```python
from build123d import *

# Parameters (mm, degrees)
SKETCH1_W                 = 79.1
SKETCH1_H                 = 60
BOSS_EXTRUDE1_DEPTH       = 5
BOSS_EXTRUDE2_DEPTH       = 24
MIRROR2_COPY_1_DEPTH      = 24
SKETCH9_W                 = 10
SKETCH9_H                 = 9.8
SKETCH9_W_2               = 6
SKETCH9_H_2               = 2.8
BOSS_EXTRUDE4_DEPTH       = 8
MIRROR9_COPY_1_SKETCH_W   = 10
MIRROR9_COPY_1_SKETCH_H   = 9.8
MIRROR9_COPY_1_SKETCH_W_2 = 6
MIRROR9_COPY_1_SKETCH_H_2 = 2.8
MIRROR9_COPY_1_DEPTH      = 8
SKETCH10_R                = 1.55
CUT_EXTRUDE6_DEPTH        = 15.8
SKETCH11_W                = 79.1
SKETCH11_H                = 16
BOSS_EXTRUDE5_DEPTH       = 16
SKETCH12_R                = 4.05
CUT_EXTRUDE7_DEPTH        = 80.1
SKETCH13_W                = 6
SKETCH13_H                = 2.8
CUT_EXTRUDE8_DEPTH        = 61
SKETCH14_R                = 1.55
CUT_EXTRUDE9_DEPTH        = 10
SKETCH14_3_W              = 6
SKETCH14_3_H              = 35
CUT_EXTRUDE10_DEPTH       = 4.8
FILLET1_R                 = 8
SKETCH15_W                = 50.3
SKETCH15_H                = 42.3
SKETCH15_R                = 1.55
SKETCH15_R_2              = 12.5
BOSS_EXTRUDE6_DEPTH       = 5
FILLET3_R                 = 3


with BuildPart() as part:
    # Sketch1 → Boss-Extrude1 (new body)
    with BuildSketch(Plane(origin=(0, 0, 0), x_dir=(1, 0, 0), z_dir=(0, 1, 0))):
        Rectangle(SKETCH1_W, SKETCH1_H)
    extrude(amount=BOSS_EXTRUDE1_DEPTH)

    # Sketch2 → Boss-Extrude2 (add)
    with BuildSketch(Plane.XY.offset(30)):
        with BuildLine():
            Line((-39.55, 13.55), (-39.55, 5))
            Line((-39.55, 5), (-20.45, 5))
            Line((-20.45, 5), (-20.45, 13.55))
            Line((-20.45, 13.55), (-22.45, 13.55))
            ThreePointArc((-22.45, 13.55), (-30, 6), (-37.55, 13.55))
            Line((-37.55, 13.55), (-39.55, 13.55))
        make_face()
    boss_extrude2 = extrude(amount=-BOSS_EXTRUDE2_DEPTH)

    # Mirror1: Boss-Extrude2 across plane
    add(boss_extrude2.mirror(Plane.XY))

    # Mirror2: Boss-Extrude2 across plane
    add(boss_extrude2.mirror(Plane(origin=(0, 0, 0), x_dir=(0, 0, 1), z_dir=(1, 0, 0))))

    # Mirror2 copy 1 sketch → Mirror2 copy 1 (add)
    with BuildSketch(Plane(origin=(0, 0, -30), x_dir=(-1, 0, 0), z_dir=(0, 0, -1))):
        with BuildLine():
            Line((-39.55, 13.55), (-39.55, 5))
            Line((-39.55, 5), (-20.45, 5))
            Line((-20.45, 5), (-20.45, 13.55))
            Line((-20.45, 13.55), (-22.45, 13.55))
            ThreePointArc((-22.45, 13.55), (-30, 6), (-37.55, 13.55))
            Line((-37.55, 13.55), (-39.55, 13.55))
        make_face()
    extrude(amount=-MIRROR2_COPY_1_DEPTH)

    # Sketch9 → Boss-Extrude4 (add)
    with BuildSketch(Plane.XY.offset(30)):
        with Locations((-15.45, 9.9)):
            Rectangle(SKETCH9_W, SKETCH9_H)
        with Locations((-15.45, 9.4)):
            Rectangle(SKETCH9_W_2, SKETCH9_H_2, mode=Mode.SUBTRACT)
    boss_extrude4 = extrude(amount=-BOSS_EXTRUDE4_DEPTH)

    # Mirror8: Boss-Extrude4 across plane
    add(boss_extrude4.mirror(Plane(origin=(0, 0, 0), x_dir=(0, 0, 1), z_dir=(1, 0, 0))))

    # Mirror9: Boss-Extrude4 across plane
    add(boss_extrude4.mirror(Plane.XY))

    # Mirror9 copy 1 sketch → Mirror9 copy 1 (add)
    with BuildSketch(Plane(origin=(0, 0, -30), x_dir=(-1, 0, 0), z_dir=(0, 0, -1))):
        with Locations((-15.45, 9.9)):
            Rectangle(MIRROR9_COPY_1_SKETCH_W, MIRROR9_COPY_1_SKETCH_H)
        with Locations((-15.45, 9.4)):
            Rectangle(MIRROR9_COPY_1_SKETCH_W_2, MIRROR9_COPY_1_SKETCH_H_2, mode=Mode.SUBTRACT)
    extrude(amount=-MIRROR9_COPY_1_DEPTH)

    # Sketch10 → Cut-Extrude6 (cut, through all)
    with BuildSketch(Plane(origin=(0, 14.8, 0), x_dir=(1, 0, 0), z_dir=(0, 1, 0))):
        with Locations(Location((-15.45, 26, 0), (0, 0, 270))):  # turned: the seam where the file's is
            Circle(SKETCH10_R)
        with Locations(Location((15.45, 26, 0), (0, 0, 270))):  # turned: the seam where the file's is
            Circle(SKETCH10_R)
        with Locations(Location((15.45, -26, 0), (0, 0, 270))):  # turned: the seam where the file's is
            Circle(SKETCH10_R)
        with Locations(Location((-15.45, -26, 0), (0, 0, 270))):  # turned: the seam where the file's is
            Circle(SKETCH10_R)
    extrude(amount=-CUT_EXTRUDE6_DEPTH, mode=Mode.SUBTRACT)

    # Sketch11 → Boss-Extrude5 (add)
    with BuildSketch(Plane.XZ):
        with Locations((0, 22)):
            Rectangle(SKETCH11_W, SKETCH11_H)
        with Locations((0, -22)):
            Rectangle(SKETCH11_W, SKETCH11_H)
    extrude(amount=BOSS_EXTRUDE5_DEPTH)

    # Sketch12 → Cut-Extrude7 (cut, through all)
    with BuildSketch(Plane(origin=(39.55, 0, 0), x_dir=(0, 0, -1), z_dir=(1, 0, 0))):
        with Locations((-22, -8)):
            Circle(SKETCH12_R)
        with Locations((22, -8)):
            Circle(SKETCH12_R)
    extrude(amount=-CUT_EXTRUDE7_DEPTH, mode=Mode.SUBTRACT)

    # Sketch13 → Cut-Extrude8 (cut, through all)
    with BuildSketch(Plane(origin=(0, 0, -30), x_dir=(-1, 0, 0), z_dir=(0, 0, -1))):
        with Locations((0, 1.6)):
            Rectangle(SKETCH13_W, SKETCH13_H)
    extrude(amount=-CUT_EXTRUDE8_DEPTH, mode=Mode.SUBTRACT)

    # Sketch14 → Cut-Extrude9 (cut)
    with BuildSketch(Plane(origin=(0, 5, 0), x_dir=(1, 0, 0), z_dir=(0, 1, 0))):
        with Locations(Location((0, -22, 0), (0, 0, 270))):  # turned: the seam where the file's is
            Circle(SKETCH14_R)
        with Locations(Location((0, 22, 0), (0, 0, 270))):  # turned: the seam where the file's is
            Circle(SKETCH14_R)
    extrude(amount=-CUT_EXTRUDE9_DEPTH, mode=Mode.SUBTRACT)

    # Sketch14_3 → Cut-Extrude10 (cut)
    with BuildSketch(Plane(origin=(0, 5, 0), x_dir=(1, 0, 0), z_dir=(0, 1, 0))):
        Rectangle(SKETCH14_3_W, SKETCH14_3_H)
    extrude(amount=-CUT_EXTRUDE10_DEPTH, mode=Mode.SUBTRACT)

    # Fillet1
    fillet1_edges = [part.edges().sort_by_distance(p)[0] for p in [
        (0, 0, -14),
        (0, 0, 14),
    ]]
    fillet(fillet1_edges, radius=FILLET1_R)

    # Sketch15 → Boss-Extrude6 (add)
    with BuildSketch(Plane.XZ):
        with Locations((-64.7, 0)):
            Rectangle(SKETCH15_W, SKETCH15_H)
        with Locations(Location((-84.2, 15.5, 0), (0, 0, 270))):  # turned: the seam where the file's is
            Circle(SKETCH15_R, mode=Mode.SUBTRACT)
        with Locations(Location((-84.2, -15.5, 0), (0, 0, 270))):  # turned: the seam where the file's is
            Circle(SKETCH15_R, mode=Mode.SUBTRACT)
        with Locations(Location((-53.2, -15.5, 0), (0, 0, 270))):  # turned: the seam where the file's is
            Circle(SKETCH15_R, mode=Mode.SUBTRACT)
        with Locations(Location((-53.2, 15.5, 0), (0, 0, 270))):  # turned: the seam where the file's is
            Circle(SKETCH15_R, mode=Mode.SUBTRACT)
        with Locations(Location((-68.7, 0, 0), (0, 0, 270))):  # turned: the seam where the file's is
            Circle(SKETCH15_R_2, mode=Mode.SUBTRACT)
    extrude(amount=-BOSS_EXTRUDE6_DEPTH)

    # Fillet3
    fillet3_edges = [part.edges().sort_by_distance(p)[0] for p in [
        (-39.55, 5, -13.575),
        (-39.55, 5, 13.575),
    ]]
    fillet(fillet3_edges, radius=FILLET3_R)


solid = part.part
```
Check sheet for the modelled part. Datum: model origin and axes. Units: mm. A direction names the side the tool comes from. Coordinates: 2 decimals unless noted, no trailing zeros. Order: outer loops, then holes, each group sorted by start corner. A loop starts at its lowest first (then second) coordinate and runs counter-clockwise, first axis right, second up. Notation, with made-up numbers: (76, 22.25) -> (129, 22.25) arc R31 cw to (129, 55.25) -> close; hole circle Ø2 at (-18.75, 38.25). An arc over 180 degrees is marked (long way). Write item = value, one per line. Start each with the question number.
1) Go/stop test with flat-tipped pins: P1, Ø5, axis at y = 8.5, z = 23, coming from the -X side; P2, Ø2.5, axis at x = 0, z = -22, coming from the +Y side; P3, Ø9.5, axis at x = -29, y = 11, coming from the +Z side; P4, Ø7, axis at x = 33, y = 10, coming from the +Z side. Record where each tip stops, or that it passes through.
2) Cross-section at C-C (x = -84.2). Enter the section's corners in (y, z).
3) Mould release check, pull along Y, two halves, no side actions. Record for faces 5 (the flat face through (-15, 0, -26)), 6 (the flat face through (0, 0.2, 0)), 7 (the cylindrical face through (-76.306, 2.465, 9.92)): +Y half, -Y half, draft (parallel to the pull), parting line (faces both ways), or undercut.
4) Cross-section at D-D (z = -15.5). State how many separate pieces and enclosed holes the cut face has, then the cut area to 3 significant figures.
5) Cross-section at A-A (x = -68.7). Enter the section's corners in (y, z), then the cut area to 3 significant figures.
6) Material ranges on L1, parallel to X at y = 13, z = 23.5; L2, parallel to X at y = 3.15, z = 15.5; L3, parallel to Z at x = -84.2, y = 1.15, recorded low to high.
7) Access from +Z, -Z, +X, -X, +Y, -Y to the whole of each face (thin tool, end or side, straight path). Record for faces 1 (the flat face through (10.45, 10, -26)), 2 (the cylindrical face through (14.075, 12.828, -25.285)), 3 (the flat face through (-1, -12, -14)), 4 (the flat face through (3, 2, 0)).
8) Cross-section at B-B (z = 0). Enter the section's corners in (x, y), then the cut area to 3 significant figures.
Ans:
q1.P1 = -39.79
q1.P2 = -11.85
q1.P3 = through
q1.P4 = 30
q2.outline = (0, -21.15) -> (5, -21.15) -> (5, -17.05) -> (0, -17.05) -> close; (0, -13.95) -> (5, -13.95) -> (5, 13.95) -> (0, 13.95) -> close; (0, 17.05) -> (5, 17.05) -> (5, 21.15) -> (0, 21.15) -> close
q3.face_5 = +Y half
q3.face_6 = undercut
q3.face_7 = draft
q4.separate_pieces = 3
q4.enclosed_holes = 0
q4.area = 2,000 mm²
q5.outline = (0, -21.15) -> (5, -21.15) -> (5, -12.5) -> (0, -12.5) -> close; (0, 12.5) -> (5, 12.5) -> (5, 21.15) -> (0, 21.15) -> close
q5.area = 86.5 mm²
q6.L1 = -39.55 to -37.53, -22.47 to -10.45, 10.45 to 22.47, 37.53 to 39.55
q6.L2 = -89.85 to -85.75, -82.65 to -54.75, -51.65 to -3, 3 to 39.55
q6.L3 = -21.15 to -17.05, -13.95 to 13.95, 17.05 to 21.15
q7.face_1 = +Z, -Z, +Y
q7.face_2 = +Y
q7.face_3 = +X, -X, -Y
q7.face_4 = none
q8.outline = (-89.85, 0) -> (-81.2, 0) -> (-81.2, 5) -> (-89.85, 5) -> close; (-56.2, 0) -> (39.55, 0) -> (39.55, 5) -> (3, 5) -> (3, 0.2) -> (-3, 0.2) -> (-3, 5) -> (-56.2, 5) -> close
q8.area = 493 mm²
